from build123d import *

# Parameters (mm, degrees)
SKETCH2_W           = 13.987360838
SKETCH2_H           = 4.9958
SKETCH2_W_2         = 13.987360839
BOSS_EXTRUDE1_DEPTH = 4.4958


with BuildPart() as part:
    # Sketch2 → Boss-Extrude1 (new body)
    with BuildSketch(Plane.ZY.offset(44.7458)):
        Polygon((5.4356, 40.058729674), (0, 40.058729674), (0, 28.740547856), (5.4356, 28.740547856), (5.4356, 16.422366038), (0, 16.422366038), (0, 5.104184219), (5.4356, 5.104184219), (5.4356, -7.213997599), (0, -7.213997599), (0, -18.532179417), (5.4356, -18.532179417), (5.4356, -32.862070326), (86.359765029, -32.862070326), (86.359765029, -18.532179417), (91.795365029, -18.532179417), (91.795365029, -7.213997599), (86.359765029, -7.213997599), (86.359765029, 5.104184219), (91.795365029, 5.104184219), (91.795365029, 16.422366038), (86.359765029, 16.422366038), (86.359765029, 28.740547856), (91.795365029, 28.740547856), (91.795365029, 40.058729674), (86.359765029, 40.058729674), align=None)
        with Locations((18.922960838, -27.189170326)):
            Rectangle(SKETCH2_W, SKETCH2_H, mode=Mode.SUBTRACT)
        with Locations((45.897682515, -27.189170326)):
            Rectangle(SKETCH2_W_2, SKETCH2_H, mode=Mode.SUBTRACT)
        with Locations((72.872404191, -27.189170326)):
            Rectangle(SKETCH2_W, SKETCH2_H, mode=Mode.SUBTRACT)
    extrude(amount=-BOSS_EXTRUDE1_DEPTH)


solid = part.part
Can you work these out from the model? Positions are in its coordinate system, mm. A direction names the side the tool comes from. Coordinates: 2 decimals unless noted, no trailing zeros. Loops run counter-clockwise (first coordinate to the right, second up) from the corner with the lowest first, then second, coordinate; pieces in that order, holes last. Notation, with made-up numbers: (42.25, 34) - (88.25, 34) arc R22 cw to (88.25, 48) - close; hole circle Ø5 at (-37.75, 34). An arc over 180 degrees is marked (long way). Answer as a JSON object with one key per item and string values. Group by question number.
Item 1: If we mould it in two halves opening along Z, with no side actions, what happens to faces 1 (the face through (-43, -24.691, 46)), 2 (the face through (-43, -13, 0)), 3 (the face through (-43, -13, 91.795))? For each: released by +Z, released by -Z, zero draft, split by the parting line, or undercut.
Item 2: If we section it at A-A (z = 42): List the corners of the cut face in (x, y) for me.
Item 3: On a 3-axis mill with a long thin cutter (end or side, diameter ignored), from which of +Z, -Z, +X, -X, +Y, -Y can I reach the whole of each face in a straight line? I mean faces 4 (the face through (-43, -27, 11.929)), 5 (the face through (-43, 5.104, 89)), 6 (the face through (-43, -7.214, 3)). Say none if no direction works.
Item 4: For pin 1 (1.5 mm diameter, centred on x = -44, y = -13.5, fed in from -Z); pin 2 (2 mm diameter, centred on x = -43, y = -27.5, fed in from -Z); pin 3 (2 mm diameter, centred on x = -43, z = 89.5, fed in from -Y), each with a flat end and sliding along its axis, tell me the tip position at first contact or that it passes through.
Item 5: If I drill on L1, parallel to Y at x = -41.8, z = 77.5; L2, parallel to Z at x = -42.05, y = 27, over which ranges is the centre line in solid material (lowest first)? Write a range as from..to.
Item 6: If we section it at B-B (x = -42.5): State how many separate pieces and enclosed holes the cut face has, plus the area to 3 significant figures.
Item 7: If we section it at C-C (y = 21): List the corners of the cut face in (x, z) for me.
Returned:
{
 "1": {"face 1": "undercut", "face 2": "released by -Z", "face 3": "released by +Z"},
 "2": {"outline": "(-44.75, -32.86) - (-40.25, -32.86) - (-40.25, -29.69) - (-44.75, -29.69) - close; (-44.75, -24.69) - (-40.25, -24.69) - (-40.25, 40.06) - (-44.75, 40.06) - close"},
 "3": {"face 4": "+X, -X", "face 5": "+Z, +X, -X", "face 6": "-Z, +X, -X"},
 "4": {"pin 1": "stops at z = 0", "pin 2": "stops at z = 5.44", "pin 3": "stops at y = -18.53"},
 "5": {"L1": "y = -32.86..-29.69, -24.69..40.06", "L2": "z = 5.44..86.36"},
 "6": {"separate pieces": "1", "enclosed holes": "3", "area": "6,060 mm²"},
 "7": {"outline": "(-44.75, 5.44) - (-40.25, 5.44) - (-40.25, 86.36) - (-44.75, 86.36) - close"}
}
